Input: dimensioned drawing with shaded views. Units: mm. Origin: part minimum x, y, z. Round coordinates to 2 decimals unless told otherwise and drop trailing zeros. Loops run counter-clockwise (first coordinate to the right, second up) from the corner with the lowest first, then second, coordinate; pieces in that order, holes last. Notation, with made-up numbers: (2, 55) - (54, 55) arc R24 cw to (54, 72) - close; hole circle Ø8 at (-9, -9). An arc over 180 degrees is marked (long way). One line per question, with ' | ' between items. Start each with the question number.
1. Ray query, line 1 (X direction, y = 0.9, z = 10); line 2 (X direction, y = 1.5, z = 39); line 3 (Z direction, x = 43.5, y = 0.3). Return the intervals inside material, ascending.
2. Pin query (flat end, axial travel): pin 1 (0.9 mm diameter, centred on x = 6, y = 1, fed in from +Z); pin 2 (13.5 mm diameter, centred on x = 36.2, z = 10, fed in from +Y). Return the tip coordinate at first contact, or that it passes through.
3. Cut plane A-A (x = 10.2). Return loops of the section in (y, z).
4. Cut plane D-D (z = 10). Return loops of the section in (x, y).
5. Cut plane B-B (z = 36.5). Return loops of the section in (x, y), then the cut area to 3 significant figures.
6. Cut plane C-C (y = 0.9). Return loops of the section in (x, z).
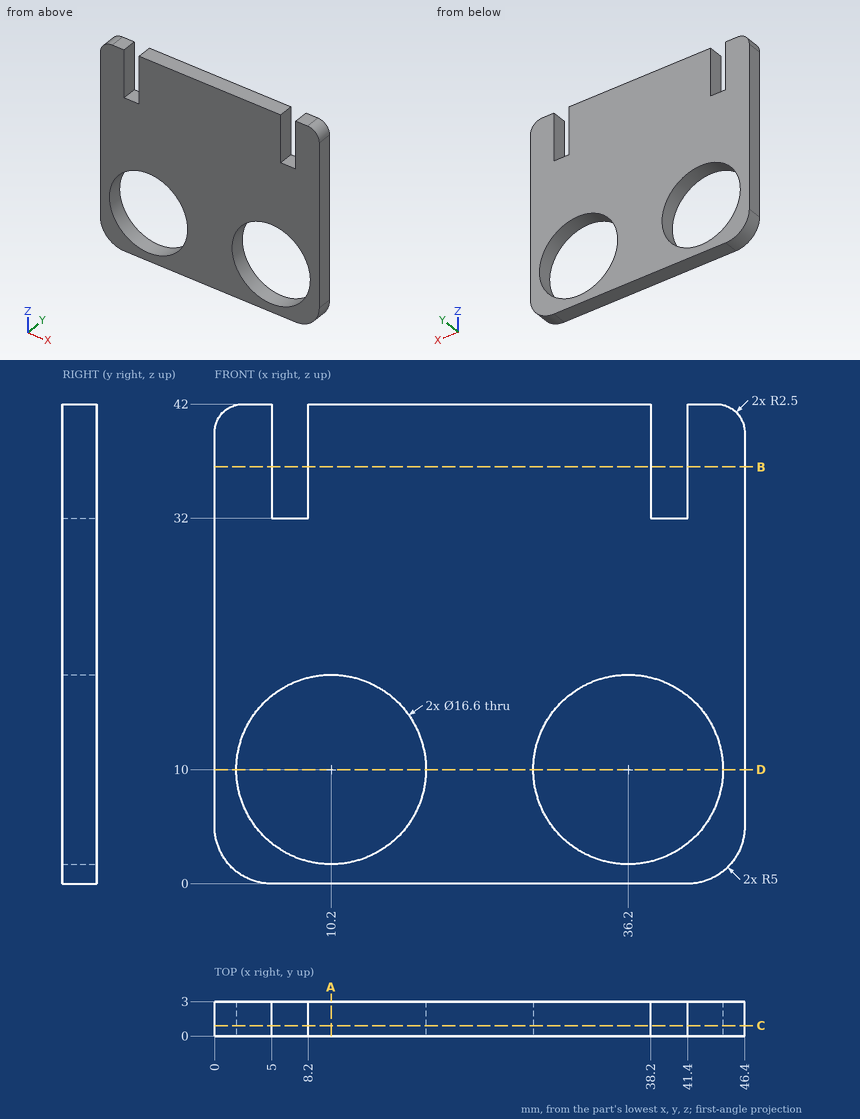
Answers follow:
1) line 1: x = 0 to 1.9, 18.5 to 27.9, 44.5 to 46.4 | line 2: x = 0 to 5, 8.2 to 38.2, 41.4 to 46.4 | line 3: z = 0.46 to 6.05, 13.95 to 42
2) pin 1: stops at z = 32 | pin 2: passes through
3) outline: (0, 0) - (3, 0) - (3, 1.7) - (0, 1.7) - close; (0, 18.3) - (3, 18.3) - (3, 42) - (0, 42) - close
4) outline: (0, 0) - (1.9, 0) - (1.9, 3) - (0, 3) - close; (18.5, 0) - (27.9, 0) - (27.9, 3) - (18.5, 3) - close; (44.5, 0) - (46.4, 0) - (46.4, 3) - (44.5, 3) - close
5) outline: (0, 0) - (5, 0) - (5, 3) - (0, 3) - close; (8.2, 0) - (38.2, 0) - (38.2, 3) - (8.2, 3) - close; (41.4, 0) - (46.4, 0) - (46.4, 3) - (41.4, 3) - close | area: 120 mm2
6) outline: (0, 5) arc R5 ccw to (5, 0) - (41.4, 0) arc R5 ccw to (46.4, 5) - (46.4, 39.5) arc R2.5 ccw to (43.9, 42) - (41.4, 42) - (41.4, 32) - (38.2, 32) - (38.2, 42) - (8.2, 42) - (8.2, 32) - (5, 32) - (5, 42) - (2.5, 42) arc R2.5 ccw to (0, 39.5) - close; hole circle Ø16.6 at (10.2, 10); hole circle Ø16.6 at (36.2, 10)
